```python
from build123d import *

# Parameters (mm, degrees)
SKETCH1_R                       = 48.5
SKETCH1_R_2                     = 1.5
BOSS_EXTRUDE1_DEPTH             = 4
SKETCH2_R                       = 3.75
CUT_EXTRUDE1_DEPTH              = 1.5
BOSS_EXTRUDE2_START             = 4
SKETCH3_R                       = 9
BOSS_EXTRUDE2_DEPTH             = 14
CUT_EXTRUDE2_START              = 6
SKETCH4_R                       = 1.25
CUT_EXTRUDE2_DEPTH              = 91.444646155
BOSS_EXTRUDE3_DEPTH             = 9
BOSS_EXTRUDE3_DIRECTION_2_REACH = 108.638


with BuildPart() as part:
    # Sketch1 → Boss-Extrude1 (new body)
    with BuildSketch(Plane(origin=(0, 0, 0), x_dir=(0, 1, 0), z_dir=(0, 0, 1))):
        with Locations(Location((0, 0, 0), (0, 0, 270))):
            Circle(SKETCH1_R)
        with Locations(Location((0, 7.25, 0), (0, 0, 270))):
            Circle(SKETCH1_R_2, mode=Mode.SUBTRACT)
        with Locations(Location((0, -7.25, 0), (0, 0, 270))):
            Circle(SKETCH1_R_2, mode=Mode.SUBTRACT)
    extrude(amount=BOSS_EXTRUDE1_DEPTH)

    # Sketch2 → Cut-Extrude1 (cut)
    with BuildSketch(Plane.XY.offset(4)):
        Circle(SKETCH2_R)
    extrude(amount=-CUT_EXTRUDE1_DEPTH, mode=Mode.SUBTRACT)

    # Sketch3 → Boss-Extrude2 (add)
    with BuildSketch(Plane(origin=(0, 0, 0), x_dir=(-1, 0, 0), z_dir=(0, 1, 0)).offset(BOSS_EXTRUDE2_START)):
        with BuildLine():
            Line((-30.34, 4), (-30.34, 11.86))
            ThreePointArc((-30.34, 11.86), (-28.924736696, 21.745164753), (-24.792654999, 30.836113728))
            Line((-24.792654999, 30.836113728), (-9.278105641, 55.104149989))
            ThreePointArc((-9.278105641, 55.104149989), (30.651097233, 62.12443475), (34.252718415, 21.743078098))
            ThreePointArc((34.252718415, 21.743078098), (31.352340729, 17.057138369), (30.34, 11.64))
            Line((30.34, 11.64), (30.34, 4))
            Line((30.34, 4), (-30.34, 4))
        make_face()
        with Locations(Location((13.91, 40.28, 0), (0, 0, 90))):
            Circle(SKETCH3_R, mode=Mode.SUBTRACT)
    extrude(amount=BOSS_EXTRUDE2_DEPTH)

    # Sketch4 → Cut-Extrude2 (cut, through all)
    with BuildSketch(Plane(origin=(0, 0, 0), x_dir=(-1, 0, 0), z_dir=(0, 1, 0)).offset(CUT_EXTRUDE2_START)):
        with Locations(Location((20.096096654, 53.537164466, 0), (0, 0, 270))):
            Circle(SKETCH4_R)
        with Locations(Location((27.167164466, 46.466096654, 0), (0, 0, 270))):
            Circle(SKETCH4_R)
        with Locations(Location((-6.773961031, 12.524971157, 0), (0, 0, 270))):
            Circle(SKETCH4_R)
        with Locations(Location((-13.845028843, 19.596038969, 0), (0, 0, 270))):
            Circle(SKETCH4_R)
        Polygon((-0.41, 11.110757595), (28.581378029, 40.102135624), (13.732135624, 54.951378029), (-15.259242405, 25.96), align=None)
    extrude(amount=CUT_EXTRUDE2_DEPTH, mode=Mode.SUBTRACT)

    # Sketch5 → Boss-Extrude3 (add)
    with BuildSketch(Plane(origin=(0, 18, 0), x_dir=(-1, 0, 0), z_dir=(0, 1, 0))):
        with BuildLine():
            Line((36.34, 4), (36.34, 11.64))
            ThreePointArc((36.34, 11.64), (36.947404437, 14.890283021), (38.687631049, 17.701846859))
            ThreePointArc((38.687631049, 17.701846859), (34.300821036, 66.886736311), (-14.333340667, 58.335960445))
            Line((-14.333340667, 58.335960445), (-29.847890025, 34.067924184))
            ThreePointArc((-29.847890025, 34.067924184), (-34.683704058, 23.428701186), (-36.34, 11.86))
            Line((-36.34, 11.86), (-36.34, 4))
            Line((-36.34, 4), (-33.34, 4))
            Line((-33.34, 4), (-30.34, 4))
            Line((-30.34, 4), (-24.79, 4))
            ThreePointArc((-24.79, 4), (-21.256686804, 30.833791886), (-9.278105641, 55.104149989))
            ThreePointArc((-9.278105641, 55.104149989), (30.651097233, 62.12443475), (34.252718415, 21.743078098))
            ThreePointArc((34.252718415, 21.743078098), (31.352340729, 17.057138369), (30.34, 11.64))
            Line((30.34, 11.64), (30.34, 4))
            Line((30.34, 4), (33.34, 4))
            Line((33.34, 4), (36.34, 4))
        make_face()
    extrude(amount=BOSS_EXTRUDE3_DEPTH)

    # Boss-Extrude3 direction 2: up to this face of the body (flat: up to its plane)
    boss_extrude3_direction_2_end = Plane(part.part.faces().sort_by_distance((-6.762869766, 4, 32.000889593))[0])
    # Sketch5 → Boss-Extrude3 direction 2 (add, up to the picked face)
    with BuildSketch(Plane(origin=(0, 18, 0), x_dir=(-1, 0, 0), z_dir=(0, 1, 0)), mode=Mode.PRIVATE) as boss_extrude3_direction_2_sk1:
        with BuildLine():
            Line((36.34, 4), (36.34, 11.64))
            ThreePointArc((36.34, 11.64), (36.947404437, 14.890283021), (38.687631049, 17.701846859))
            ThreePointArc((38.687631049, 17.701846859), (34.300821036, 66.886736311), (-14.333340667, 58.335960445))
            Line((-14.333340667, 58.335960445), (-29.847890025, 34.067924184))
            ThreePointArc((-29.847890025, 34.067924184), (-34.683704058, 23.428701186), (-36.34, 11.86))
            Line((-36.34, 11.86), (-36.34, 4))
            Line((-36.34, 4), (-33.34, 4))
            Line((-33.34, 4), (-30.34, 4))
            Line((-30.34, 4), (-24.79, 4))
            ThreePointArc((-24.79, 4), (-21.256686804, 30.833791886), (-9.278105641, 55.104149989))
            ThreePointArc((-9.278105641, 55.104149989), (30.651097233, 62.12443475), (34.252718415, 21.743078098))
            ThreePointArc((34.252718415, 21.743078098), (31.352340729, 17.057138369), (30.34, 11.64))
            Line((30.34, 11.64), (30.34, 4))
            Line((30.34, 4), (33.34, 4))
            Line((33.34, 4), (36.34, 4))
        make_face()
    boss_extrude3_direction_2_tool1 = split(extrude(boss_extrude3_direction_2_sk1.sketch, amount=-BOSS_EXTRUDE3_DIRECTION_2_REACH, mode=Mode.PRIVATE), bisect_by=boss_extrude3_direction_2_end, keep=Keep.BOTH, mode=Mode.PRIVATE)
    add(boss_extrude3_direction_2_tool1.solids().sort_by(Axis((-35.249588, 18, 7.82), (0, -1, 0)))[0])


solid = part.part
```
Work out the finished part from the listing and answer in its coordinate system (mm). A direction names the side the tool comes from. Round coordinates to 2 decimals unless told otherwise and drop trailing zeros. Write each loop counter-clockwise with the first axis right and the second up, starting at its lowest first coordinate (ties: lowest second). Pieces come first, ordered by that corner, then holes. Notation, with made-up numbers: (-39, 13.25) - (-24, 13.25) arc R25 cw to (-24, 45.25) - close; hole circle Ø4 at (-5.5, 28.25). An arc over 180 degrees is marked (long way). Return JSON: item names as keys, results as strings. Group by question number.
Q1. The part is cut by section C-C on z = 66.5. Write down the section's boundary in (x, y), then the cut area to 3 significant figures.
Q2. The mould has two halves that part along Y. Classify faces 5 (the cylindrical face through (14.32, 11.92, 18.44)), 6 (the cylindrical face through (-3.746, 0.165, 3.26)), 7 (the flat face through (7, 6, 13)): released by +Y, released by -Y, zero draft, split by the parting line, or undercut.
Q3. The part is cut by section A-A on y = 0. Write down the section's boundary in (x, z).
Q4. For faces 1 (the flat face through (13.3, 27, 49.4)), 2 (the flat face through (-36.34, 16, 8)), 3 (the flat face through (21.982, 15.661, 46.372)), 4 (the cylindrical face through (-20.94, 11.92, 54.46)), determine the directions among +Z, -Z, +X, -X, +Y, -Y from which every point of the face is accessible in a straight line to the end or side of a thin tool.
Q5. The part is cut by section B-B on z = 43.5. Write down the section's boundary in (x, y), then the cut area to 3 significant figures.
Q6. Each of these flat-tipped pins is pushed along its axis until it touches: pin 1 Ø6 at (y, z) = (20.5, 9) entering from +X; pin 2 Ø21 at (x, z) = (1.5, 22.5) entering from -Y; pin 3 Ø5 at (x, y) = (-3.5, -13) entering from +Z. Where does it stop, or does it pass through?
Q7. Find the intervals of material crossed by L1, parallel to Z at x = 10.5, y = 10; L2, parallel to Y at x = 0, z = 3.55; L3, parallel to Z at x = -16, y = -12.5, in increasing order.
Q8. The part is cut by section D-D on z = 36. Write down the section's boundary in (x, y).
Solved:
{
 "1": {"outline": "(-34.8, 4) - (6.98, 4) - (6.98, 27) - (-5.55, 27) - (-5.55, 18) - (-22.27, 18) - (-22.27, 27) - (-34.8, 27) - close", "area": "810 mm²"},
 "2": {"face 5": "zero draft", "face 6": "undercut", "face 7": "released by +Y"},
 "3": {"outline": "(-48.5, 0) - (-8.75, 0) - (-8.75, 4) - (-48.5, 4) - close; (-5.75, 0) - (5.75, 0) - (5.75, 4) - (3.75, 4) - (3.75, 2.5) - (-3.75, 2.5) - (-3.75, 4) - (-5.75, 4) - close; (8.75, 0) - (48.5, 0) - (48.5, 4) - (8.75, 4) - close"},
 "4": {"face 1": "+Z, +X, -X, +Y", "face 2": "-X, +Y, -Y", "face 3": "+Z, +X, +Y, -Y", "face 4": "+Y"},
 "5": {"outline": "(-47.28, 4) - (-22.31, 4) - (-22.31, 6) - (-25.18, 6) - (-25.18, 18) - (-41.24, 18) - (-41.24, 27) - (-47.28, 27) - close; (-5.51, 4) - (23.82, 4) - (23.82, 27) - (16.24, 27) - (16.24, 18) - (-2.28, 18) - (-2.28, 6) - (-5.51, 6) - close", "area": "809 mm²"},
 "6": {"pin 1": "x = 36.34", "pin 2": "y = 4", "pin 3": "z = 4"},
 "7": {"L1": "0 to 21.2, 30.72 to 53.19, 53.35 to 63.26", "L2": "-48.5 to -3.75, 3.75 to 48.5", "L3": "0 to 4"},
 "8": {"outline": "(-47.16, 4) - (-21.83, 4) - (-21.83, 6) - (-24.48, 6) - (-24.48, 18) - (-41.1, 18) - (-41.1, 27) - (-47.16, 27) - close; (-5.99, 4) - (28.61, 4) - (28.61, 27) - (19.5, 27) - (19.5, 18) - (5.22, 18) - (5.22, 6) - (-5.99, 6) - close"}
}
